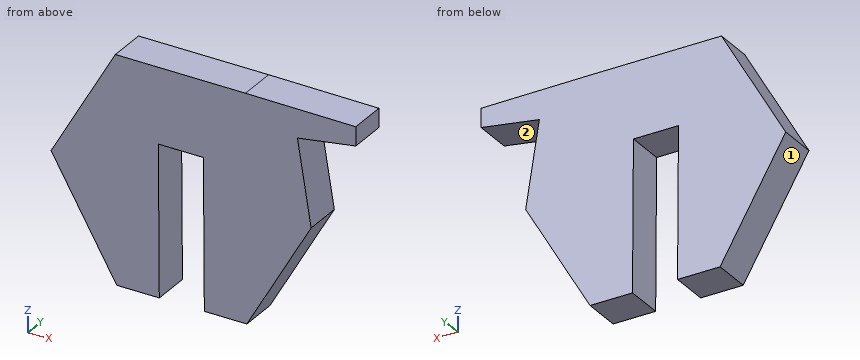
from build123d import *

# Parameters (mm, degrees)
BOSS_EXTRUDE1_DEPTH = 2.5
SKETCH2_W           = 3
SKETCH2_H           = 2.5
CUT_EXTRUDE1_DEPTH  = 10


with BuildPart() as part:
    # Sketch1 → Boss-Extrude1 (new body)
    with BuildSketch(Plane(origin=(0, 0, 0), x_dir=(1, 0, 0), z_dir=(0, 1, 0))):
        Polygon((12.694105225, -6.934131302), (12.694105225, -8.188855223), (5.34603962, -8.188855223), (-3.3140449, -8.134669239), (-7.59716072, -0.607723054), (-3.220192022, 6.865037146), (5.439892498, 6.810851162), (9.723008318, -0.716095023), (8.810324475, -6.299245302), align=None)
    extrude(amount=BOSS_EXTRUDE1_DEPTH)

    # Sketch2 → Cut-Extrude1 (cut)
    with BuildSketch(Plane(origin=(0.04282666, 0, -6.8446205), x_dir=(-0.999980426, 0, -0.006256859), z_dir=(0.006256859, 0, -0.999980426))):
        with Locations((-1.067171483, 1.25)):
            Rectangle(SKETCH2_W, SKETCH2_H)
    extrude(amount=-CUT_EXTRUDE1_DEPTH, mode=Mode.SUBTRACT)


solid = part.part
Work out the finished part from the listing and answer in its coordinate system (mm). Face numbers are marked on the shaded views. A direction names the side the tool comes from. Give positions to 0.01 mm unless a question says otherwise; leave off trailing zeros. Write each loop counter-clockwise with the first axis right and the second up, starting at its lowest first coordinate (ties: lowest second). Pieces come first, ordered by that corner, then holes. Notation, with made-up numbers: (7.25, -37) - (63.25, -37) arc R25 ccw to (63.25, -12) - close; hole circle Ø3 at (22.25, 4). An arc over 180 degrees is marked (long way). One line per item, written item: value. Start each with the question number.
1. For the marked faces 1 and 2, determine the directions among +Z, -Z, +X, -X, +Y, -Y from which every point of the face is accessible in a straight line to the end or side of a thin tool.
2. Find section A-A (z = -4). Write down the section's boundary in (x, y).
3. Given pin 1 (1 mm diameter, centred on y = 1, z = 1.5, fed in from -X); pin 2 (1.5 mm diameter, centred on y = 2, z = -3, fed in from +X), each flat-ended and moving along its own axis, determine where each tip first touches the part or whether it passes through.
4. Find section B-B (y = 0.55). Write down the section's boundary in (x, z), then the cut area to 3 significant figures.
5. Find section C-C (z = 2.25). Write down the section's boundary in (x, y).
6. Find section D-D (x = 1.5). Write down the section's boundary in (y, z), then the cut area to 3 significant figures.
7. Consider probe 1 along X at (y, z) = (1.7, -4.5); probe 2 along Z at (x, y) = (5.25, 2); probe 3 along X at (y, z) = (0.55, 0.75). Determine where each line is inside the solid, lowest interval first.
Geometry results:
1. face 1: -Z, -X, +Y, -Y
1. face 2: +X, +Y, -Y
2. outline: (-4.9, 0) - (-0.41, 0) - (-0.41, 2.5) - (-4.9, 2.5) - close; (2.59, 0) - (7.04, 0) - (7.04, 2.5) - (2.59, 2.5) - close
3. pin 1: x = -7.37
3. pin 2: x = 8.04
4. outline: (-7.6, 0.61) - (-3.22, -6.87) - (-0.39, -6.85) - (-0.45, 3.15) - (2.55, 3.17) - (2.61, -6.83) - (5.44, -6.81) - (9.72, 0.72) - (8.81, 6.3) - (12.69, 6.93) - (12.69, 8.19) - (5.35, 8.19) - (-3.31, 8.13) - close
4. area: 183 mm2
5. outline: (-6.66, 0) - (-0.45, 0) - (-0.45, 2.5) - (-6.66, 2.5) - close; (2.55, 0) - (9.47, 0) - (9.47, 2.5) - (2.55, 2.5) - close
6. outline: (0, 3.16) - (2.5, 3.16) - (2.5, 8.16) - (0, 8.16) - close
6. area: 12.5 mm2
7. probe 1: -4.61 to -0.4, 2.6 to 6.75
7. probe 2: -6.81 to 8.19
7. probe 3: -7.52 to -0.44, 2.56 to 9.72
